Job drawing, mm, ordinate dimensions from the low corner. One solid piece. A direction names the side the tool comes from. Coordinates: 2 decimals unless noted, no trailing zeros. Loops run counter-clockwise (first coordinate to the right, second up) from the corner with the lowest first, then second, coordinate; pieces in that order, holes last. Notation, with made-up numbers: (46, 62.5) - (87, 62.5) arc R20 ccw to (87, 90.5) - close; hole circle Ø3 at (11, 83). An arc over 180 degrees is marked (long way). Use a Markdown table: item, result. Add a question column.
1. Band-saw the part on B-B, the plane x = 44.5. Give the cut face in (y, z), plus the area to 3 significant figures.
2. Band-saw the part on D-D, the plane y = 16.5. Give the cut face in (x, z), plus the area to 3 significant figures.
3. Band-saw the part on C-C, the plane z = 4.25. Give the cut face in (x, y), plus the area to 3 significant figures.
4. Wall check: probe 1 along Y at (x, z) = (129, 0.3); probe 2 along Y at (x, z) = (0.9, 8); probe 3 along X at (y, z) = (8.5, 3.5). Give the ranges that are in metal, low to high. Write a range as [from, to].
5. Band-saw the part on A-A, the plane y = 39. Give the cut face in (x, z), plus the area to 3 significant figures.
6. Pull direction Y, two halves, no side cores. Call the marked faces 3, 4, 5 and 6: pulls with the +Y half, pulls with the -Y half, needs draft (parallel to the pull), parting line crosses it, or undercut.
7. 3-axis set-ups, long thin cutter, end or side, ignore diameter. For the marked faces 1 and 2: which of +Z, -Z, +X, -X, +Y, -Y reach the whole face in a straight line?
8. Drop flat-ended pins along their axis: pin 1 (5 mm diameter, centred on x = 129, y = 39, fed in from +Z); pin 2 (0.5 mm diameter, centred on x = 134.5, y = 7.5, fed in from +Z); pin 3 (12 mm diameter, centred on y = 24.5, z = 13, fed in from +X). Give the stop position or say it passes through.
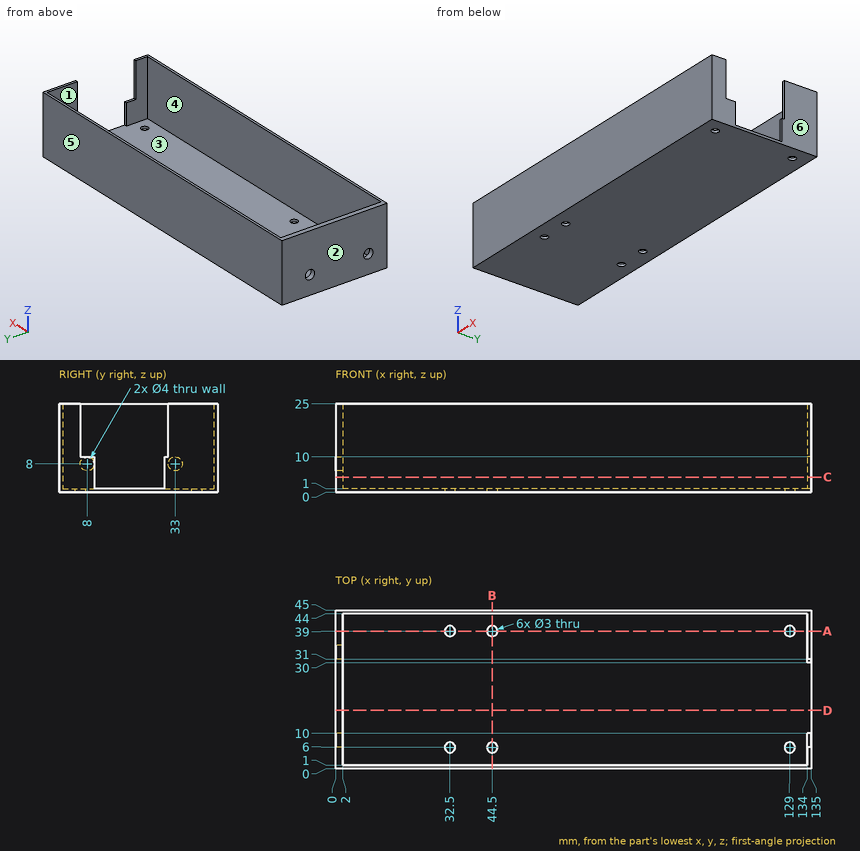
Geometry check:
| question | item | result |
|---|---|---|
| 1 | outline | (0, 0) - (4.5, 0) - (4.5, 1) - (1, 1) - (1, 25) - (0, 25) - close; (7.5, 0) - (37.5, 0) - (37.5, 1) - (7.5, 1) - close; (40.5, 0) - (45, 0) - (45, 25) - (44, 25) - (44, 1) - (40.5, 1) - close |
| 1 | area | 87.0 mm^2 |
| 2 | outline | (0, 0) - (135, 0) - (135, 1) - (2, 1) - (2, 25) - (0, 25) - close |
| 2 | area | 183 mm^2 |
| 3 | outline | (0, 0) - (135, 0) - (135, 10) - (134, 10) - (134, 1) - (2, 1) - (2, 44) - (134, 44) - (134, 30) - (135, 30) - (135, 45) - (0, 45) - close |
| 3 | area | 379 mm^2 |
| 4 | probe 1 | y = [0, 4.5], [7.5, 37.5], [40.5, 45] |
| 4 | probe 2 | y = [0, 6], [10, 31], [35, 45] |
| 4 | probe 3 | x = [0, 2], [134, 135] |
| 5 | outline | (0, 0) - (31, 0) - (31, 1) - (2, 1) - (2, 25) - (0, 25) - close; (34, 0) - (43, 0) - (43, 1) - (34, 1) - close; (46, 0) - (127.5, 0) - (127.5, 1) - (46, 1) - close; (130.5, 0) - (135, 0) - (135, 25) - (134, 25) - (134, 1) - (130.5, 1) - close |
| 5 | area | 198 mm^2 |
| 6 | face 3 | undercut |
| 6 | face 4 | undercut |
| 6 | face 5 | pulls with the +Y half |
| 6 | face 6 | needs draft |
| 7 | face 1 | +Z |
| 7 | face 2 | +Z, -Z, -X, +Y, -Y |
| 8 | pin 1 | stops at z = 1 |
| 8 | pin 2 | stops at z = 10 |
| 8 | pin 3 | stops at x = 2 |
